Here's the drawing with two shaded views (mm, measured from the low corner). I have some questions. Give positions to 0.01 mm unless a question says otherwise; leave off trailing zeros. Write each loop counter-clockwise with the first axis right and the second up, starting at its lowest first coordinate (ties: lowest second). Pieces come first, ordered by that corner, then holes. Notation, with made-up numbers: (8, 13) - (26, 13) arc R21 ccw to (26, 45) - close; hole circle Ø6 at (18.25, 0). An arc over 180 degrees is marked (long way). Answer as CSV lines item,"result". Start each with the question number.
Q1. Imagine slicing it at B-B on z = 47.5. List the corners of the cut face in (x, y) for me.
Q2. Imagine slicing it at C-C on x = 258. List the corners of the cut face in (y, z) for me, and give its area (4 significant figures).
Q3. If I drill on line 1 along X through (y, z) = (2.25, 259); line 2 along Z through (x, y) = (235.5, 5.5); line 3 along Z through (x, y) = (117.5, 2.25), over which ranges is the centre line in solid material (lowest first)?
Q4. Imagine slicing it at A-A on y = 4.5. List the corners of the cut face in (x, z) for me, and give its area (3 significant figures).
Q5. Will these pins go through, and if not, where does the flat tip stop? pin 1 Ø2 at (x, y) = (132.5, 4.5) entering from +Z; pin 2 Ø3 at (x, y) = (255, 1.5) entering from +Z; pin 3 Ø1.9 at (x, y) = (258.5, 4.5) entering from -Z.
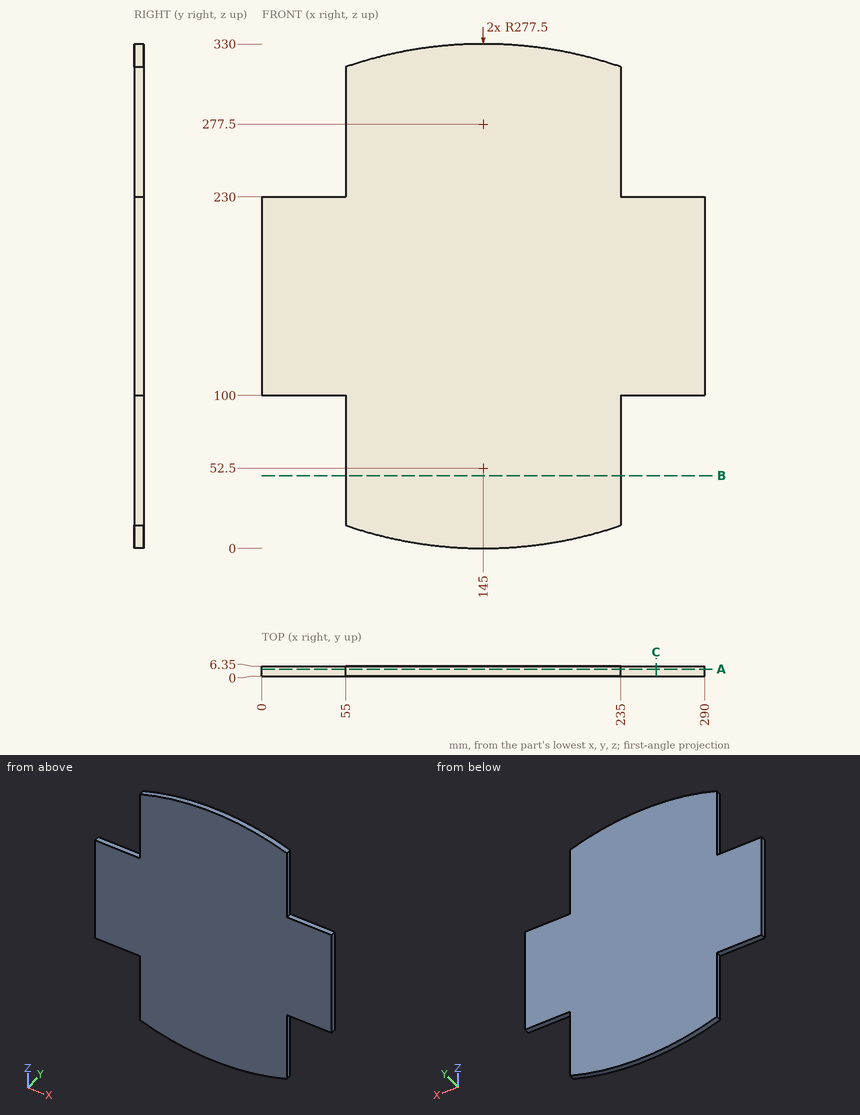
Conclusion:
1,outline,"(55, 0) - (235, 0) - (235, 6.35) - (55, 6.35) - close"
2,outline,"(0, 100) - (6.35, 100) - (6.35, 230) - (0, 230) - close"
2,area,"825.5 mm^2"
3,line 1,"55 to 235"
3,line 2,"100 to 230"
3,line 3,"1.37 to 328.63"
4,outline,"(0, 100) - (55, 100) - (55, 15) arc R277.5 ccw to (235, 15) - (235, 100) - (290, 100) - (290, 230) - (235, 230) - (235, 315) arc R277.5 ccw to (55, 315) - (55, 230) - (0, 230) - close"
4,area,"71,900 mm^2"
5,pin 1,"z = 329.76"
5,pin 2,"z = 230"
5,pin 3,"z = 100"
